Part model, mm, in its own coordinate system. Face numbers are marked on the shaded views. A direction names the side the tool comes from. Give positions to 0.01 mm unless a question says otherwise; leave off trailing zeros. Write each loop counter-clockwise with the first axis right and the second up, starting at its lowest first coordinate (ties: lowest second). Pieces come first, ordered by that corner, then holes. Notation, with made-up numbers: M -31.5,-9 L 23.5,-9 A22 ccw 23.5,7 Z; hole C 59,86 d1. An arc over 180 degrees is marked long. Use CSV: the item, a comma, the result in double quotes. Start each with the question number.
Item 1: Mould opens along X. For the marked faces 3 and 4 say: released by +X, released by -X, zero draft, split by the parting line, or undercut.
Item 2: Which spindle directions (+Z, -Z, +X, -X, +Y, -Y) get a long thin tool onto all of the face, cutting with end or side? Do the marked faces 1 and 2. Say none if no direction does.
Item 3: Cut at A-A (y = 29.56). List the corners of the cut face in (x, z).
Item 4: Cut at C-C (z = 0.9). List the corners of the cut face in (x, y).
Item 5: Cut at B-B (x = 29.56). List the corners of the cut face in (y, z), then the cut area to 3 significant figures.
Item 6: Drill centre lines: line 1 (Y direction, x = 29.56, z = 3.1); line 2 (X direction, y = 12, z = 3); line 3 (X direction, y = 21, z = 2.45). Where is each one in solid material? Low to high. Write a range as [from, to].
Item 7: Pin check, flat tips, straight feed: pin 1 (1.5 mm diameter, centred on y = 24.5, z = 2.5, fed in from -X); pin 2 (1.3 mm diameter, centred on x = 40, y = 26.5, fed in from +Z). Stop position of each tip, or through.
Item 8: Cut at D-D (y = 20). List the corners of the cut face in (x, z), then the cut area to 3 significant figures.
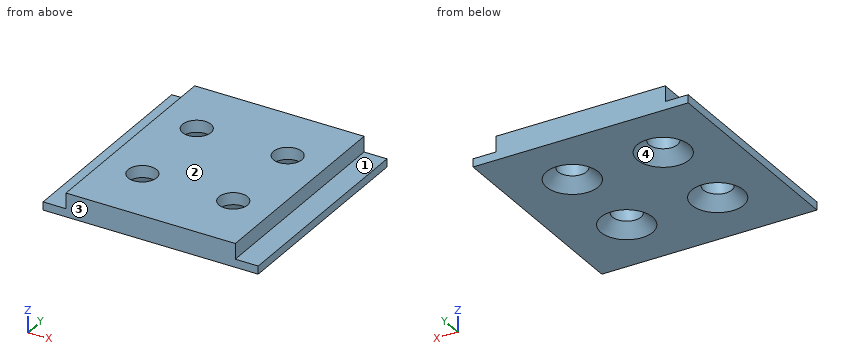
from build123d import *

# Parameters (mm, degrees)
F0_W           = 41.56
F0_H           = 41.56
F1_DEPTH       = 1.56
F2_W           = 32.7
F2_H           = 41.56
F3_DEPTH       = 3
F5_D           = 5.5
F5_DEPTH       = 8
F5_CSINK_D     = 10
F5_CSINK_ANGLE = 90


with BuildPart() as f1:
    # F0 (on Top) → F1 (new body)
    with BuildSketch(Plane.XY):
        with Locations((20.78, 20.78)):
            Rectangle(F0_W, F0_H)
    extrude(amount=F1_DEPTH)

    # F2 (on face) → F3 (join)
    with BuildSketch(Plane.XY.offset(1.56)):
        with Locations((20.78, 20.78)):
            Rectangle(F2_W, F2_H)
    extrude(amount=F3_DEPTH)

    # F5
    with Locations(Plane(origin=(0, 0, 0), x_dir=(1, 0, 0), z_dir=(0, 0, -1))):
        with Locations((12, -12), (29.56, -12), (12, -29.56), (29.56, -29.56)):
            CounterSinkHole(F5_D / 2, F5_CSINK_D / 2, depth=F5_DEPTH, counter_sink_angle=F5_CSINK_ANGLE)


solid = f1.part
Worked answers:
1,face 3,"zero draft"
1,face 4,"undercut"
2,face 1,"+Z, +X, +Y, -Y"
2,face 2,"+Z, +X, -X, +Y, -Y"
3,outline,"M 0,0 L 7,0 L 9.25,2.25 L 9.25,4.56 L 4.43,4.56 L 4.43,1.56 L 0,1.56 Z; M 14.75,2.25 L 17,0 L 24.56,0 L 26.81,2.25 L 26.81,4.56 L 14.75,4.56 Z; M 32.31,2.25 L 34.56,0 L 41.56,0 L 41.56,1.56 L 37.13,1.56 L 37.13,4.56 L 32.31,4.56 Z"
4,outline,"M 0,0 L 41.56,0 L 41.56,41.56 L 0,41.56 Z; hole C 12,12 d8.2; hole C 12,29.56 d8.2; hole C 29.56,12 d8.2; hole C 29.56,29.56 d8.2"
5,outline,"M 0,0 L 7,0 L 9.25,2.25 L 9.25,4.56 L 0,4.56 Z; M 14.75,2.25 L 17,0 L 24.56,0 L 26.81,2.25 L 26.81,4.56 L 14.75,4.56 Z; M 32.31,2.25 L 34.56,0 L 41.56,0 L 41.56,4.56 L 32.31,4.56 Z"
5,area,"129 mm^2"
6,line 1,"y = [0, 9.25], [14.75, 26.81], [32.31, 41.56]"
6,line 2,"x = [4.43, 9.25], [14.75, 26.81], [32.31, 37.13]"
6,line 3,"x = [4.43, 37.13]"
7,pin 1,"stops at x = 4.43"
7,pin 2,"stops at z = 1.56"
8,outline,"M 0,0 L 41.56,0 L 41.56,1.56 L 37.13,1.56 L 37.13,4.56 L 4.43,4.56 L 4.43,1.56 L 0,1.56 Z"
8,area,"163 mm^2"
